Verification items for the finished model (mm, model axes). A direction names the side the tool comes from. Coordinates: 2 decimals unless noted, no trailing zeros. Loops run counter-clockwise (first coordinate to the right, second up) from the corner with the lowest first, then second, coordinate; pieces in that order, holes last.
Q1. Material ranges on probe 1 along Y at (x, z) = (451, -42.5); probe 2 along Z at (x, y) = (450, 93.25); probe 3 along Z at (x, y) = (450, 28.5), recorded low to high.
Q2. Access from +Z, -Z, +X, -X, +Y, -Y to the whole of each face (thin tool, end or side, straight path). Record for faces 5 (the face through (456, -22.5, -41)), 6 (the face through (457.3, 61, -42.8)), 7 (the face through (444, 76.5, -54)), 8 (the face through (458, 90, -47)).
Q3. Sectioned sample at B-B (x = 450). Count the separate pieces of the cut face and the enclosed holes in it, then the cut area to 3 significant figures.
Q4. Go/stop test with flat-tipped pins: P1, Ø3, axis at x = 449, z = -48, coming from the -Y side; P2, Ø1.5, axis at x = 455, y = 7, coming from the +Z side; P3, Ø1.2, axis at y = 4, z = -51, coming from the +X side; P4, Ø1.7, axis at x = 450, z = -46, coming from the +Y side. Record where each tip stops, or that it passes through.
Q5. Sectioned sample at A-A (y = 31). Enter the section's corners in (x, z), then the cut area to 3 significant figures.
Q6. Mould release check, pull along Z, two halves, no side actions. Record for faces 1 (the face through (450, -29, -50)), 2 (the face through (452.43, 75.79, -47.77)), 3 (the face through (457.669, -17.974, -47.105)), 4 (the face through (456, 60.2, -54.1)): +Z half, -Z half, draft (parallel to the pull), parting line (faces both ways), or undercut.
```python
from build123d import *

# Parameters (mm, degrees)
CYLINDER547_R     = 1.5
CYLINDER547_DEPTH = 6
BOX342_W          = 20
BOX342_H          = 128
BOX342_DEPTH      = 1
BOX341_W          = 20
BOX341_H          = 128
BOX341_DEPTH      = 1
CYLINDER149_R     = 2.8
CYLINDER149_DEPTH = 25
CYLINDER150_R     = 2.8
CYLINDER150_DEPTH = 25
CYLINDER541_R     = 1.75
CYLINDER541_DEPTH = 15
CYLINDER540_R     = 1.75
CYLINDER540_DEPTH = 15
CYLINDER542_R     = 1.75
CYLINDER542_DEPTH = 15
CYLINDER543_R     = 1.75
CYLINDER543_DEPTH = 15
CYLINDER151_R     = 1.25
CYLINDER151_DEPTH = 10
CYLINDER548_R     = 1.25
CYLINDER548_DEPTH = 10
CYLINDER549_R     = 1.25
CYLINDER549_DEPTH = 10
CYLINDER550_R     = 1.25
CYLINDER550_DEPTH = 10
CYLINDER545_R     = 5.6
CYLINDER545_DEPTH = 4
CYLINDER546_R     = 5.6
CYLINDER546_DEPTH = 4
CYLINDER544_R     = 2.55
CYLINDER544_DEPTH = 128
BOX343_W          = 5.5
BOX343_H          = 6
BOX343_DEPTH      = 15
BOX344_W          = 5.5
BOX344_H          = 6
BOX344_DEPTH      = 15
FILLET132_R       = 2
BOX340_W          = 20
BOX340_H          = 8
BOX340_DEPTH      = 15
FILLET131_R       = 3
BOX339_W          = 20
BOX339_H          = 8
BOX339_DEPTH      = 15
FILLET130_R       = 3
CYLINDER142_R     = 8
CYLINDER142_DEPTH = 128


with BuildPart() as cylinder642:
    # Cylinder547 → Cylinder547 (new body)
    with BuildSketch(Plane.XY.offset(-7.5)):
        Circle(CYLINDER547_R)
    extrude(amount=CYLINDER547_DEPTH)


with BuildPart() as cube413:
    # Box342 → Box342 (new body)
    with BuildSketch(Plane(origin=(-10, -64, 7.5), x_dir=(1, 0, 0), z_dir=(0, 0, 1))):
        with Locations((10, 64)):
            Rectangle(BOX342_W, BOX342_H)
    extrude(amount=BOX342_DEPTH)


with BuildPart() as fusion127:
    # Box341 → Box341 (new body)
    with BuildSketch(Plane(origin=(-10, -64, -8.5), x_dir=(1, 0, 0), z_dir=(0, 0, 1))):
        with Locations((10, 64)):
            Rectangle(BOX341_W, BOX341_H)
    extrude(amount=BOX341_DEPTH)

    # Fusion127: union Cube413
    add(cube413.part)


with BuildPart() as cylinder149:
    # Cylinder149 → Cylinder149 (new body)
    with BuildSketch(Plane(origin=(0, -30, 0), x_dir=(1, 0, 0), z_dir=(0, 1, 0))):
        Circle(CYLINDER149_R)
    extrude(amount=CYLINDER149_DEPTH)


with BuildPart() as fusion465:
    # Cylinder150 → Cylinder150 (new body)
    with BuildSketch(Plane(origin=(0, 5, 0), x_dir=(1, 0, 0), z_dir=(0, 1, 0))):
        Circle(CYLINDER150_R)
    extrude(amount=CYLINDER150_DEPTH)

    # Fusion465: union Cylinder149
    add(cylinder149.part)


with BuildPart() as cylinder636:
    # Cylinder541 → Cylinder541 (new body)
    with BuildSketch(Plane(origin=(13.5, -49.5, 13), x_dir=(1, 0, 0), z_dir=(0, 0, 1))):
        Circle(CYLINDER541_R)
    extrude(amount=CYLINDER541_DEPTH)


with BuildPart() as fusion461:
    # Cylinder540 → Cylinder540 (new body)
    with BuildSketch(Plane(origin=(13.5, 49.5, 13), x_dir=(1, 0, 0), z_dir=(0, 0, 1))):
        Circle(CYLINDER540_R)
    extrude(amount=CYLINDER540_DEPTH)

    # Fusion461: union Cylinder636
    add(cylinder636.part)


with BuildPart() as cylinder637:
    # Cylinder542 → Cylinder542 (new body)
    with BuildSketch(Plane(origin=(13.5, -49.5, 13), x_dir=(1, 0, 0), z_dir=(0, 0, 1))):
        Circle(CYLINDER542_R)
    extrude(amount=CYLINDER542_DEPTH)


with BuildPart() as fusion463:
    # Cylinder543 → Cylinder543 (new body)
    with BuildSketch(Plane(origin=(13.5, 49.5, 13), x_dir=(1, 0, 0), z_dir=(0, 0, 1))):
        Circle(CYLINDER543_R)
    extrude(amount=CYLINDER543_DEPTH)

    # Fusion462: union Cylinder637
    add(cylinder637.part)


with BuildPart() as fusion463_1:
    # Fusion462 placement: moved
    add(fusion463.part.moved(Location((-12, 0, 0))))

    # Fusion463: union Fusion461
    add(fusion461.part)


with BuildPart() as fusion463_2:
    # Fusion463 placement: moved
    add(fusion463_1.part.moved(Location((-7.5, 0, -20.5))))


with BuildPart() as cylinder151:
    # Cylinder151 → Cylinder151 (new body)
    with BuildSketch(Plane(origin=(0, -27, 4.5), x_dir=(0, 0, -1), z_dir=(1, 0, 0))):
        Circle(CYLINDER151_R)
    extrude(amount=CYLINDER151_DEPTH)


with BuildPart() as fusion468:
    # Cylinder548 → Cylinder548 (new body)
    with BuildSketch(Plane(origin=(0, -27, -4.5), x_dir=(0, 0, -1), z_dir=(1, 0, 0))):
        Circle(CYLINDER548_R)
    extrude(amount=CYLINDER548_DEPTH)

    # Fusion468: union Cylinder151
    add(cylinder151.part)


with BuildPart() as cylinder644:
    # Cylinder549 → Cylinder549 (new body)
    with BuildSketch(Plane(origin=(0, -27, 4.5), x_dir=(0, 0, -1), z_dir=(1, 0, 0))):
        Circle(CYLINDER549_R)
    extrude(amount=CYLINDER549_DEPTH)


with BuildPart() as fusion470:
    # Cylinder550 → Cylinder550 (new body)
    with BuildSketch(Plane(origin=(0, -27, -4.5), x_dir=(0, 0, -1), z_dir=(1, 0, 0))):
        Circle(CYLINDER550_R)
    extrude(amount=CYLINDER550_DEPTH)

    # Fusion469: union Cylinder644
    add(cylinder644.part)


with BuildPart() as fusion470_1:
    # Fusion469 placement: moved
    add(fusion470.part.moved(Location((0, 54, 0))))

    # Fusion470: union Fusion468
    add(fusion468.part)


with BuildPart() as fusion470_2:
    # Fusion470 placement: moved
    add(fusion470_1.part.moved(Location((-2, 0, 0))))


with BuildPart() as cylinder640:
    # Cylinder545 → Cylinder545 (new body)
    with BuildSketch(Plane(origin=(0, -64, 0), x_dir=(1, 0, 0), z_dir=(0, 1, 0))):
        Circle(CYLINDER545_R)
    extrude(amount=CYLINDER545_DEPTH)


with BuildPart() as fusion124:
    # Cylinder546 → Cylinder546 (new body)
    with BuildSketch(Plane(origin=(0, 60, 0), x_dir=(1, 0, 0), z_dir=(0, 1, 0))):
        Circle(CYLINDER546_R)
    extrude(amount=CYLINDER546_DEPTH)

    # Fusion124: union Cylinder640
    add(cylinder640.part)


with BuildPart() as fusion464:
    # Cylinder544 → Cylinder544 (new body)
    with BuildSketch(Plane(origin=(0, -64, 0), x_dir=(1, 0, 0), z_dir=(0, 1, 0))):
        Circle(CYLINDER544_R)
    extrude(amount=CYLINDER544_DEPTH)

    # Fusion464: union Fusion124
    add(fusion124.part)


with BuildPart() as cube414:
    # Box343 → Box343 (new body)
    with BuildSketch(Plane(origin=(2.5, -30, -7.5), x_dir=(1, 0, 0), z_dir=(0, 0, 1))):
        with Locations((2.75, 3)):
            Rectangle(BOX343_W, BOX343_H)
    extrude(amount=BOX343_DEPTH)


with BuildPart() as fillet132:
    # Box344 → Box344 (new body)
    with BuildSketch(Plane(origin=(2.5, 24, -7.5), x_dir=(1, 0, 0), z_dir=(0, 0, 1))):
        with Locations((2.75, 3)):
            Rectangle(BOX344_W, BOX344_H)
    extrude(amount=BOX344_DEPTH)

    # Fusion466: union Cube414
    add(cube414.part)

    # Fillet132
    fillet132_edges = [fillet132.edges().sort_by_distance(p)[0] for p in [
        (5.25, 24, -7.5),
        (5.25, 24, 7.5),
        (5.25, 30, -7.5),
        (5.25, 30, 7.5),
        (5.25, -30, -7.5),
        (5.25, -30, 7.5),
        (5.25, -24, -7.5),
        (5.25, -24, 7.5),
    ]]
    fillet(fillet132_edges, radius=FILLET132_R)


with BuildPart() as fillet131:
    # Box340 → Box340 (new body)
    with BuildSketch(Plane(origin=(-10, -53.5, -7.5), x_dir=(1, 0, 0), z_dir=(0, 0, 1))):
        with Locations((10, 4)):
            Rectangle(BOX340_W, BOX340_H)
    extrude(amount=BOX340_DEPTH)

    # Fillet131
    fillet131_edges = [fillet131.edges().sort_by_distance(p)[0] for p in [
        (-10, -53.5, 0),
        (-10, -45.5, 0),
        (10, -53.5, 0),
        (10, -45.5, 0),
    ]]
    fillet(fillet131_edges, radius=FILLET131_R)


with BuildPart() as fillet130:
    # Box339 → Box339 (new body)
    with BuildSketch(Plane(origin=(-10, -53.5, -7.5), x_dir=(1, 0, 0), z_dir=(0, 0, 1))):
        with Locations((10, 4)):
            Rectangle(BOX339_W, BOX339_H)
    extrude(amount=BOX339_DEPTH)

    # Fillet130
    fillet130_edges = [fillet130.edges().sort_by_distance(p)[0] for p in [
        (-10, -53.5, 0),
        (-10, -45.5, 0),
        (10, -53.5, 0),
        (10, -45.5, 0),
    ]]
    fillet(fillet130_edges, radius=FILLET130_R)


with BuildPart() as fillet130_1:
    # Fillet130 placement: moved
    add(fillet130.part.moved(Location((0, 99, 0))))


with BuildPart() as axle_front_wide:
    # Cylinder142 → Cylinder142 (new body)
    with BuildSketch(Plane(origin=(0, -64, 0), x_dir=(1, 0, 0), z_dir=(0, 1, 0))):
        Circle(CYLINDER142_R)
    extrude(amount=CYLINDER142_DEPTH)

    # Fusion126: union Fillet131, Fillet130
    add(fillet131.part)
    add(fillet130_1.part)

    # Fusion467: union Fillet132
    add(fillet132.part)

    # Cut359: cut Fusion464
    add(fusion464.part, mode=Mode.SUBTRACT)

    # Cut360: cut Fusion470
    add(fusion470_2.part, mode=Mode.SUBTRACT)

    # Cut047: cut Fusion463
    add(fusion463_2.part, mode=Mode.SUBTRACT)

    # Cut048: cut Fusion465
    add(fusion465.part, mode=Mode.SUBTRACT)

    # Cut049: cut Fusion127
    add(fusion127.part, mode=Mode.SUBTRACT)

    # Cut050: cut Cylinder642
    add(cylinder642.part, mode=Mode.SUBTRACT)


with BuildPart() as axle_front_wide_1:
    # Cut050 placement: moved
    add(axle_front_wide.part.moved(Location((450, 31, -47))))


solid = axle_front_wide_1.part
```
Geometry check:
1. probe 1: y = -29 to 2.75, 5.25 to 56.75, 59.25 to 91
1. probe 2: z = -54.5 to -52.6, -41.4 to -39.5
1. probe 3: z = -54.5 to -49.55, -44.45 to -39.5
2. face 5: +Z, +X, -Y
2. face 6: +Z, +X
2. face 7: -Z, -X
2. face 8: +X, +Y
3. separate pieces: 3
3. enclosed holes: 4
3. area: 1,160 mm2
4. P1: stops at y = -29
4. P2: stops at z = -39.94
4. P3: stops at x = 448
4. P4: passes through
5. outline: (447.22, -54.5) - (448.5, -54.5) - (448.5, -49.06) arc R2.55 cw (long way) to (451.5, -49.06) - (451.5, -54.5) - (452.78, -54.5) arc R8 ccw to (452.78, -39.5) - (447.22, -39.5) arc R8 ccw to start
5. area: 162 mm2
6. face 1: undercut
6. face 2: undercut
6. face 3: draft
6. face 4: -Z half
